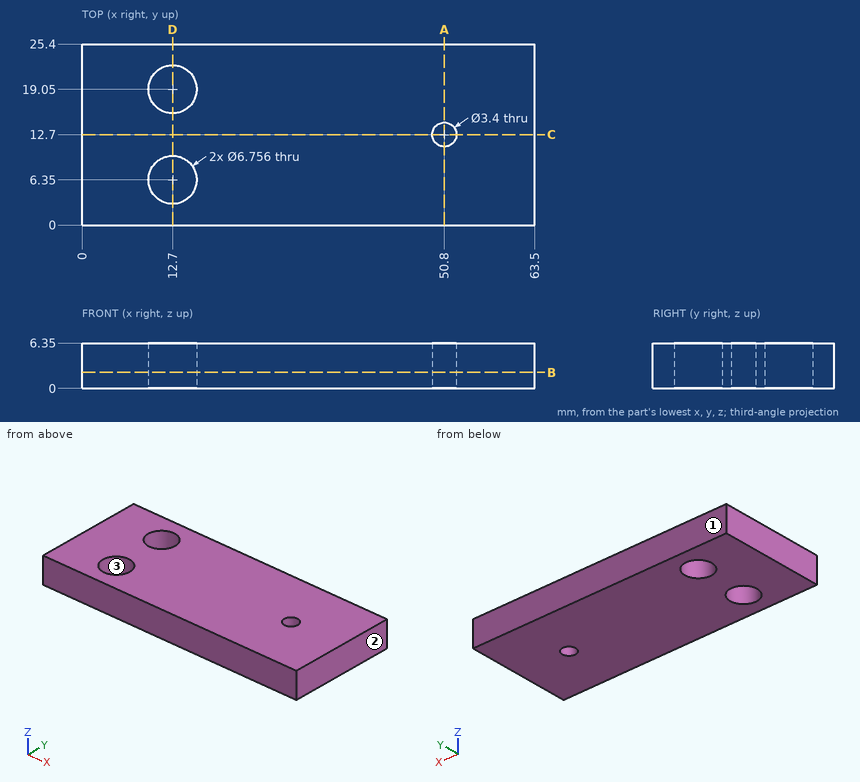
Geometry check sheet. Reference: drawing and pictorial views, mm from the part's lowest x, y, z. Round coordinates to 2 decimals unless told otherwise and drop trailing zeros. Loops run counter-clockwise (first coordinate to the right, second up) from the corner with the lowest first, then second, coordinate; pieces in that order, holes last. Notation, with made-up numbers: (50.25, -12.75) - (109.25, -12.75) arc R21 cw to (109.25, -1.75) - close; hole circle Ø10 at (-22.5, 84). An arc over 180 degrees is marked (long way). Write item = value, one per line. Start each with the question number.
Q1. Section check C-C (y = 12.7). Record the boundary of the cut face in (x, z), plus the area to 3 significant figures.
Q2. Thickness scan on L1, parallel to Y at x = 12.7, z = 3.75; L2, parallel to Y at x = 50.8, z = 2.75; L3, parallel to Y at x = 14, z = 3.5. Record the ranges inside material, lowest first.
Q3. Release check for a two-part mould opening along X. For the marked faces 1, 2 and 3 record: pulls with the +X half, pulls with the -X half, needs draft (parallel to the pull), parting line crosses it, or undercut.
Q4. Section check B-B (z = 2.25). Record the boundary of the cut face in (x, y), plus the area to 3 significant figures.
Q5. Section check D-D (x = 12.7). Record the boundary of the cut face in (y, z).
Q6. Section check A-A (x = 50.8). Record the boundary of the cut face in (y, z).
Derived:
q1.outline = (0, 0) - (49.1, 0) - (49.1, 6.35) - (0, 6.35) - close; (52.5, 0) - (63.5, 0) - (63.5, 6.35) - (52.5, 6.35) - close
q1.area = 382 mm^2
q2.L1 = 0 to 2.97, 9.73 to 15.67, 22.43 to 25.4
q2.L2 = 0 to 11, 14.4 to 25.4
q2.L3 = 0 to 3.23, 9.47 to 15.93, 22.17 to 25.4
q3.face_1 = needs draft
q3.face_2 = pulls with the +X half
q3.face_3 = undercut
q4.outline = (0, 0) - (63.5, 0) - (63.5, 25.4) - (0, 25.4) - close; hole circle Ø6.76 at (12.7, 6.35); hole circle Ø6.76 at (12.7, 19.05); hole circle Ø3.4 at (50.8, 12.7)
q4.area = 1,530 mm^2
q5.outline = (0, 0) - (2.97, 0) - (2.97, 6.35) - (0, 6.35) - close; (9.73, 0) - (15.67, 0) - (15.67, 6.35) - (9.73, 6.35) - close; (22.43, 0) - (25.4, 0) - (25.4, 6.35) - (22.43, 6.35) - close
q6.outline = (0, 0) - (11, 0) - (11, 6.35) - (0, 6.35) - close; (14.4, 0) - (25.4, 0) - (25.4, 6.35) - (14.4, 6.35) - close
